Answer from the drawing. Dimensions are ordinates in mm from the lowest x, y and z of the part. Coordinates: 2 decimals unless noted, no trailing zeros. Write each loop counter-clockwise with the first axis right and the second up, starting at its lowest first coordinate (ties: lowest second). Pieces come first, ordered by that corner, then holes. Notation, with made-up numbers: (58, 34.5) -> (87, 34.5) arc R26 ccw to (87, 72.5) -> close; hole circle Ø10 at (21, -0.75). An arc over 180 degrees is marked (long way). Answer as a JSON object with one key per item and string values. Group by question number.
(1) Find section B-B (z = 11.5). Give the vertices of the cut face in (x, y) (3 decimals), then the cut area to 3 significant figures.
(2) Find section C-C (y = 381). Give the vertices of the cut face in (x, z) (3 decimals).
(3) Find section A-A (x = 25.4). Give the vertices of the cut face in (y, z) (3 decimals).
(4) Find section D-D (y = 27). Give the vertices of the cut face in (x, z).
(5) Straight lines are drawn through the part: L1, parallel to Y at x = 25.4, z = 14.5 (3 decimals); L2, parallel to Y at x = 87, z = 8.25; L3, parallel to X at y = 52.5, z = 14.5. For each, find the intervals that lie inside material, in ascending order.
(6) Flat-ended cylindrical pins translate along their axes: P1, Ø8, axis at x = 236, y = 89, coming from the -Z side; P2, Ø9.5, axis at y = 189.5, z = 7, coming from the -X side; P3, Ø4, axis at x = 139.5, z = 3, coming from the +Y side; P4, Ø5, axis at y = 324.5, z = 10.5, coming from the +X side. Find the tip coordinate at first contact, or state that the pin passes through.
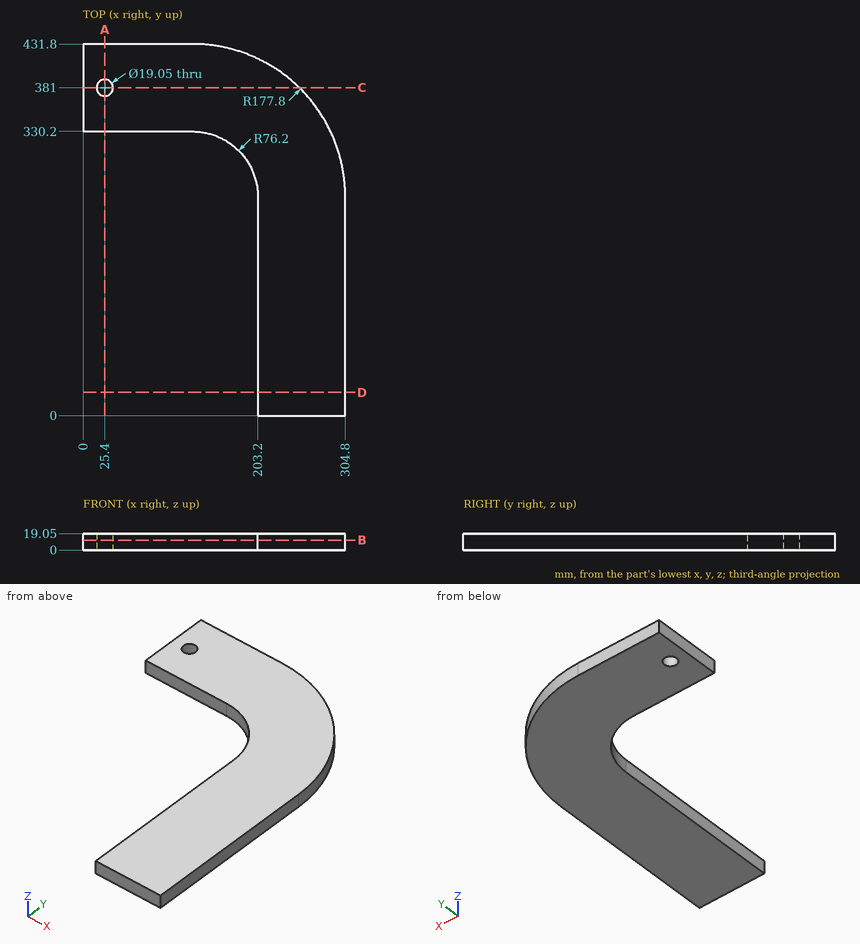
Results below:
{
 "1": {"outline": "(0, 330.2) -> (127, 330.2) arc R76.2 cw to (203.2, 254) -> (203.2, 0) -> (304.8, 0) -> (304.8, 254) arc R177.8 ccw to (127, 431.8) -> (0, 431.8) -> close; hole circle Ø19.05 at (25.4, 381)", "area": "58,700 mm2"},
 "2": {"outline": "(0, 0) -> (15.875, 0) -> (15.875, 19.05) -> (0, 19.05) -> close; (34.925, 0) -> (251.434, 0) -> (251.434, 19.05) -> (34.925, 19.05) -> close"},
 "3": {"outline": "(330.2, 0) -> (371.475, 0) -> (371.475, 19.05) -> (330.2, 19.05) -> close; (390.525, 0) -> (431.8, 0) -> (431.8, 19.05) -> (390.525, 19.05) -> close"},
 "4": {"outline": "(203.2, 0) -> (304.8, 0) -> (304.8, 19.05) -> (203.2, 19.05) -> close"},
 "5": {"L1": "y = 330.2 to 371.475, 390.525 to 431.8", "L2": "y = 330.2 to 431.8", "L3": "x = 203.2 to 304.8"},
 "6": {"P1": "stops at z = 0", "P2": "stops at x = 203.2", "P3": "stops at y = 431.49", "P4": "stops at x = 291.28"}
}
